Could you check a few things on this model? Use its own coordinates, in mm. Round coordinates to 2 decimals unless told otherwise and drop trailing zeros. Write each loop counter-clockwise with the first axis right and the second up, starting at its lowest first coordinate (ties: lowest second). Pieces come first, ordered by that corner, then holes. Notation, with made-up numbers: (-37.75, 88.25) -> (-5.75, 88.25) arc R8 ccw to (-5.75, 98.25) -> close; hole circle Ø9 at (85, 85.25). An arc over 180 degrees is marked (long way). Answer in a Markdown table with one row per item. Add a question column.
```python
from build123d import *

# Parameters (mm, degrees)
SKETCH1_W           = 50
SKETCH1_H           = 80
SKETCH1_R           = 2.5
BOSS_EXTRUDE1_DEPTH = 11.5


with BuildPart() as part:
    # Sketch1 → Boss-Extrude1 (new body)
    with BuildSketch(Plane.XY):
        Polygon((-161.5, 350), (-161.5, -350), (-81.5, -350), (161.5, -350), (161.5, 350), align=None)
        with Locations((77.5, 143.5)):
            Rectangle(SKETCH1_W, SKETCH1_H, mode=Mode.SUBTRACT)
        with BuildLine():
            ThreePointArc((-81.5, -89.5), (-79, -92), (-81.5, -94.5))
            ThreePointArc((-81.5, -94.5), (-84, -92), (-81.5, -89.5))
        make_face(mode=Mode.SUBTRACT)
        with Locations((-81.5, -62)):
            Circle(SKETCH1_R, mode=Mode.SUBTRACT)
        with Locations((-41.5, 30)):
            Circle(SKETCH1_R, mode=Mode.SUBTRACT)
    extrude(amount=BOSS_EXTRUDE1_DEPTH)


solid = part.part
```
(1) Suppose I cut it at A-A, the plane x = 65. Please give me the cut outline in (y, z).
(2) I need wall thicknesses on L1, parallel to Y at x = -81.5, z = 5.5; L2, parallel to Y at x = -41.5, z = 7.75; L3, parallel to Y at x = 93, z = 1.5. Which ranges of each line are inside material? Lowest first, please.
(3) Suppose I cut it at B-B, the plane z = 9.5. Please give me the cut outline in (x, y), then the cut area to 3 significant figures.
Response:
| question | item | result |
|---|---|---|
| 1 | outline | (-350, 0) -> (103.5, 0) -> (103.5, 11.5) -> (-350, 11.5) -> close; (183.5, 0) -> (350, 0) -> (350, 11.5) -> (183.5, 11.5) -> close |
| 2 | L1 | -350 to -94.5, -89.5 to -64.5, -59.5 to 350 |
| 2 | L2 | -350 to 27.5, 32.5 to 350 |
| 2 | L3 | -350 to 103.5, 183.5 to 350 |
| 3 | outline | (-161.5, -350) -> (161.5, -350) -> (161.5, 350) -> (-161.5, 350) -> close; hole circle Ø5 at (-81.5, -92); hole circle Ø5 at (-81.5, -62); hole circle Ø5 at (-41.5, 30); hole (52.5, 103.5) -> (102.5, 103.5) -> (102.5, 183.5) -> (52.5, 183.5) -> close |
| 3 | area | 222,000 mm² |
